Study the drawing (mm; zero at the part's minimum x, y, z) and answer. A direction names the side the tool comes from. Give positions to 0.01 mm unless a question says otherwise; leave off trailing zeros. Loops run counter-clockwise (first coordinate to the right, second up) from the corner with the lowest first, then second, coordinate; pieces in that order, holes last. Notation, with made-up numbers: (-14.5, 10) - (9.5, 10) arc R16 cw to (9.5, 33) - close; hole circle Ø11 at (87, 1). An arc over 180 degrees is marked (long way). Answer in a Markdown table with one row per item. Add a question column.
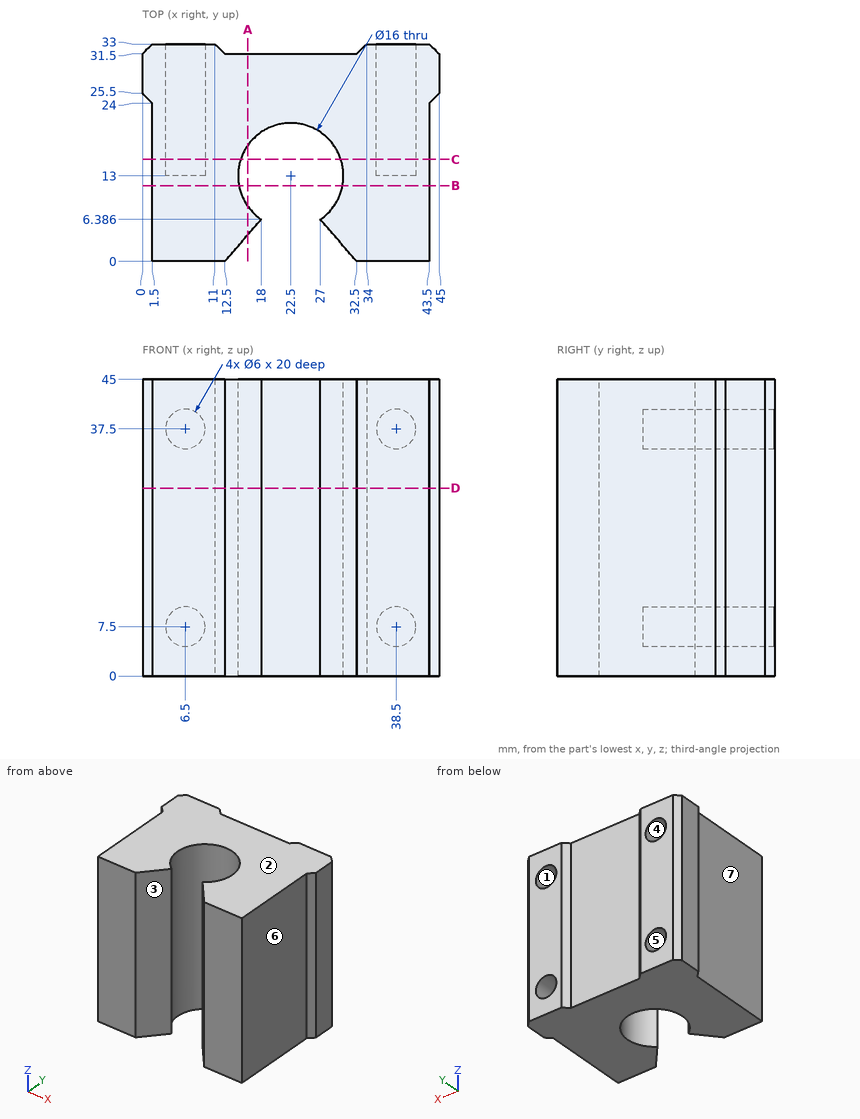
(1) Find the intervals of material crossed by line 1 along Z through (x, y) = (38.5, 21.25); line 2 along X through (y, z) = (13, 18); line 3 along X through (y, z) = (25, 37), in increasing order. Write a range as [from, to].
(2) Given pin 1 Ø3 at (y, z) = (3.5, 39) entering from +X; pin 2 Ø8 at (x, y) = (21.5, 13) entering from +Z; pin 3 Ø10 at (y, z) = (3.5, 25) entering from -X; pin 4 Ø1.8 at (x, z) = (39, 38.5) entering from +Y, each flat-ended and moving along its own axis, determine where each tip first touches the part or whether it passes through.
(3) A cutting plane is placed at C-C on y = 15.5. Determine the outline of the cut face in (x, z), plus the area to 3 significant figures.
(4) A cutting plane is placed at A-A on x = 16. Determine the outline of the cut face in (y, z).
(5) The mould has two halves that part along Z. Classify the marked faces 1, 2, 3 and 4: pulls with the +Z half, pulls with the -Z half, needs draft (parallel to the pull), parting line crosses it, or undercut.
(6) A cutting plane is placed at D-D on z = 28.5. Determine the outline of the cut face in (x, y) (1 decimal), plus the area to 3 significant figures.
(7) A cutting plane is placed at B-B on y = 11.5. Determine the outline of the cut face in (x, z).
(8) A tool of negligible diameter and unlimited length cuts with its end or side. For the marked faces 5, 6 and 7, from which of +Z, -Z, +X, -X, +Y, -Y can it reach the whole face along a straight path? Write none if from no direction.
Evaluation:
| question | item | result |
|---|---|---|
| 1 | line 1 | z = [0, 4.5], [10.5, 34.5], [40.5, 45] |
| 1 | line 2 | x = [1.5, 14.5], [30.5, 43.5] |
| 1 | line 3 | x = [0.5, 3.54], [9.46, 35.54], [41.46, 44.5] |
| 2 | pin 1 | stops at x = 43.5 |
| 2 | pin 2 | passes through |
| 2 | pin 3 | stops at x = 1.5 |
| 2 | pin 4 | stops at y = 13 |
| 3 | outline | (1.5, 0) - (14.9, 0) - (14.9, 45) - (1.5, 45) - close; (30.1, 0) - (43.5, 0) - (43.5, 45) - (30.1, 45) - close; hole circle Ø6 at (6.5, 7.5); hole circle Ø6 at (6.5, 37.5); hole circle Ø6 at (38.5, 7.5); hole circle Ø6 at (38.5, 37.5) |
| 3 | area | 1,090 mm² |
| 4 | outline | (4.06, 0) - (8.34, 0) - (8.34, 45) - (4.06, 45) - close; (17.66, 0) - (31.5, 0) - (31.5, 45) - (17.66, 45) - close |
| 5 | face 1 | undercut |
| 5 | face 2 | pulls with the +Z half |
| 5 | face 3 | needs draft |
| 5 | face 4 | undercut |
| 6 | outline | (0, 25.5) - (1.5, 24) - (1.5, 0) - (12.5, 0) - (18, 6.4) arc R8 cw (long way) to (27, 6.4) - (32.5, 0) - (43.5, 0) - (43.5, 24) - (45, 25.5) - (45, 31.5) - (43.5, 33) - (34, 33) - (32.5, 31.5) - (12.5, 31.5) - (11, 33) - (1.5, 33) - (0, 31.5) - close |
| 6 | area | 1,090 mm² |
| 7 | outline | (1.5, 0) - (14.64, 0) - (14.64, 45) - (1.5, 45) - close; (30.36, 0) - (43.5, 0) - (43.5, 45) - (30.36, 45) - close |
| 8 | face 5 | +Y |
| 8 | face 6 | +Z, -Z, +X, -Y |
| 8 | face 7 | +Z, -Z, -X, -Y |
